Input: part model. Units: mm. Frame: model coordinates. A direction names the side the tool comes from. Round coordinates to 2 decimals unless told otherwise and drop trailing zeros. Loops run counter-clockwise (first coordinate to the right, second up) from the corner with the lowest first, then second, coordinate; pieces in that order, holes last. Notation, with made-up numbers: (29.25, 10.5) -> (87.25, 10.5) arc R11 ccw to (87.25, 21.5) -> close; hole circle Ø5 at (72, 19). An arc over 180 degrees is marked (long way). Answer as a JSON object with one key per item and string values.
```python
from build123d import *

# Parameters (mm, degrees)
F0_W      = 40.93
F0_H      = 16.6
F0_W_2    = 7.73
F0_H_2    = 7.73
F0_W_3    = 10.6
F0_H_3    = 10.6
F0_R      = 4
F0_W_4    = 6.33
F0_H_4    = 6.33
F1_DEPTH  = 2
F2_W      = 40.93
F2_H      = 16.6
F2_W_2    = 11.6
F2_H_2    = 12.6
F2_W_3    = 7.73
F2_H_3    = 7.73
F3_DEPTH  = 15
F4_W      = 40.93
F4_H      = 16.6
F4_W_2    = 11.6
F4_H_2    = 12.6
F4_W_3    = 7.73
F4_H_3    = 7.73
F5_DEPTH  = 0.5
F7_DEPTH  = 4
F8_R      = 3.5
F9_DEPTH  = 3
F10_R     = 3.5
F11_DEPTH = 3


with BuildPart() as f1:
    # F0 (on Top) → F1 (new body)
    with BuildSketch(Plane.XY):
        Rectangle(F0_W, F0_H)
        Polygon((-6.865, 6.3), (-6.865, 6.865), (6.865, 6.865), (6.865, 6.3), (18.465, 6.3), (18.465, -6.3), (6.865, -6.3), (6.865, -6.865), (-6.865, -6.865), (-6.865, -6.3), (-18.465, -6.3), (-18.465, 6.3), align=None, mode=Mode.SUBTRACT)
        Polygon((6.865, 6.865), (-6.865, 6.865), (-6.865, 6.3), (-6.865, 5.3), (-6.865, -5.3), (-6.865, -6.3), (-6.865, -6.865), (6.865, -6.865), (6.865, -6.3), (6.865, -5.3), (6.865, 5.3), (6.865, 6.3), align=None)
        Rectangle(F0_W_2, F0_H_2, mode=Mode.SUBTRACT)
        with Locations((12.165, 0)):
            Rectangle(F0_W_3, F0_H_3)
        with Locations((12.165, 0)):
            Circle(F0_R, mode=Mode.SUBTRACT)
        with Locations((-12.165, 0)):
            Rectangle(F0_W_3, F0_H_3)
        with Locations((-12.165, 0)):
            Circle(F0_R, mode=Mode.SUBTRACT)
        Rectangle(F0_W_2, F0_H_2)
        Rectangle(F0_W_4, F0_H_4, mode=Mode.SUBTRACT)
        Rectangle(F0_W_4, F0_H_4)
        Polygon((-6.865, 5.3), (-6.865, 6.3), (-18.465, 6.3), (-18.465, -6.3), (-6.865, -6.3), (-6.865, -5.3), (-17.465, -5.3), (-17.465, 5.3), align=None)
        Polygon((18.465, 6.3), (6.865, 6.3), (6.865, 5.3), (17.465, 5.3), (17.465, -5.3), (6.865, -5.3), (6.865, -6.3), (18.465, -6.3), align=None)
    extrude(amount=F1_DEPTH)

    # F2 (on face) → F3 (join)
    with BuildSketch(Plane.XY.offset(2)):
        Rectangle(F2_W, F2_H)
        with Locations((-12.665, 0)):
            Rectangle(F2_W_2, F2_H_2, mode=Mode.SUBTRACT)
        Rectangle(F2_W_3, F2_H_3, mode=Mode.SUBTRACT)
        with Locations((12.665, 0)):
            Rectangle(F2_W_2, F2_H_2, mode=Mode.SUBTRACT)
    extrude(amount=F3_DEPTH)

    # F4 (on face) → F5 (join)
    with BuildSketch(Plane.XY.offset(17)):
        Rectangle(F4_W, F4_H)
        with Locations((-12.665, 0)):
            Rectangle(F4_W_2, F4_H_2, mode=Mode.SUBTRACT)
        Rectangle(F4_W_3, F4_H_3, mode=Mode.SUBTRACT)
        with Locations((12.665, 0)):
            Rectangle(F4_W_2, F4_H_2, mode=Mode.SUBTRACT)
        Rectangle(F4_W_3, F4_H_3)
    extrude(amount=F5_DEPTH)

    # F6 (on face) → F7 (cut)
    with BuildSketch(Plane.YZ.offset(6.865)):
        Polygon((0, 9.4), (-3.4, 9.4), (-3.4, 2.6), (3.4, 2.6), (3.4, 9.4), align=None)
    extrude(amount=-F7_DEPTH, mode=Mode.SUBTRACT)

    # F8 (on face) → F9 (cut)
    with BuildSketch(Plane(origin=(0, 8.3, 0), x_dir=(-1, 0, 0), z_dir=(0, 1, 0))):
        with Locations((-12.665, 13.5)):
            Circle(F8_R)
    extrude(amount=-F9_DEPTH, mode=Mode.SUBTRACT)

    # F10 (on face) → F11 (cut)
    with BuildSketch(Plane.XZ.offset(8.3)):
        with Locations((-12.665, 13.5)):
            Circle(F10_R)
    extrude(amount=-F11_DEPTH, mode=Mode.SUBTRACT)


solid = f1.part
```
1) Section A-A, the plane y = 0. Output: boundary loops of the cut face in (x, z) (3 decimals), plus the area to 3 significant figures.
Output:
{"outline": "(-20.465, 0) -> (-16.165, 0) -> (-16.165, 2) -> (-18.465, 2) -> (-18.465, 17.5) -> (-20.465, 17.5) -> close; (-8.165, 0) -> (8.165, 0) -> (8.165, 2) -> (6.865, 2) -> (6.865, 2.6) -> (3.865, 2.6) -> (3.865, 2) -> (-3.865, 2) -> (-3.865, 17) -> (3.865, 17) -> (3.865, 9.4) -> (6.865, 9.4) -> (6.865, 17.5) -> (-6.865, 17.5) -> (-6.865, 2) -> (-8.165, 2) -> close; (16.165, 0) -> (20.465, 0) -> (20.465, 17.5) -> (18.465, 17.5) -> (18.465, 2) -> (16.165, 2) -> close", "area": "188 mm^2"}
2) Section C-C, the plane x = -2. Output: boundary loops of the cut face in (y, z) (3 decimals), plus the area to 3 significant figures.
Output:
{"outline": "(-8.3, 0) -> (8.3, 0) -> (8.3, 17.5) -> (-8.3, 17.5) -> close; hole (-3.865, 2) -> (3.865, 2) -> (3.865, 17) -> (-3.865, 17) -> close", "area": "175 mm^2"}
3) Section D-D, the plane z = 13.5. Output: boundary loops of the cut face in (x, y) (3 decimals).
Output:
{"outline": "(-20.465, -8.3) -> (-16.165, -8.3) -> (-16.165, -6.3) -> (-18.465, -6.3) -> (-18.465, 6.3) -> (-6.865, 6.3) -> (-6.865, -6.3) -> (-9.165, -6.3) -> (-9.165, -8.3) -> (20.465, -8.3) -> (20.465, 8.3) -> (16.165, 8.3) -> (16.165, 6.3) -> (18.465, 6.3) -> (18.465, -6.3) -> (6.865, -6.3) -> (6.865, 6.3) -> (9.165, 6.3) -> (9.165, 8.3) -> (-20.465, 8.3) -> close; hole (-3.865, -3.865) -> (3.865, -3.865) -> (3.865, 3.865) -> (-3.865, 3.865) -> close"}
4) Draft query along Y for faces 4 (the face through (5, -3.4, 6)), 5 (the face through (-17, 0, 2)), 6 (the face through (0, 8.3, 9)), 7 (the face through (0, 0, 0)). Return one class per face: +Y half, -Y half, draft (parallel to the pull), parting line (faces both ways), or undercut.
Output:
{"face 4": "undercut", "face 5": "undercut", "face 6": "+Y half", "face 7": "draft"}
5) Ray query, probe 1 along X at (y, z) = (4.5, 16) (3 decimals); probe 2 along X at (y, z) = (1.5, 13.5) (3 decimals); probe 3 along X at (y, z) = (2.5, 3.75) (3 decimals). Return the intervals inside material, ascending.
Output:
{"probe 1": "x = -20.465 to -18.465, -6.865 to 6.865, 18.465 to 20.465", "probe 2": "x = -20.465 to -18.465, -6.865 to -3.865, 3.865 to 6.865, 18.465 to 20.465", "probe 3": "x = -20.465 to -18.465, -6.865 to -3.865, 18.465 to 20.465"}
6) Contact query for flat-ended pins moving along their axis: P1, Ø6, axis at x = 14.5, y = 1, coming from the +Z side; P2, Ø4, axis at x = -12.665, z = 13.5, coming from the -Y side. Output: stop coordinate, or through.
Output:
{"P1": "stops at z = 2", "P2": "stops at y = 6.3"}
7) Section B-B, the plane z = 9. Output: boundary loops of the cut face in (x, y) (3 decimals).
Output:
{"outline": "(-20.465, -8.3) -> (20.465, -8.3) -> (20.465, 8.3) -> (-20.465, 8.3) -> close; hole (-18.465, -6.3) -> (-6.865, -6.3) -> (-6.865, 6.3) -> (-18.465, 6.3) -> close; hole (-3.865, -3.865) -> (3.865, -3.865) -> (3.865, -3.4) -> (6.865, -3.4) -> (6.865, -6.3) -> (18.465, -6.3) -> (18.465, 6.3) -> (6.865, 6.3) -> (6.865, 3.4) -> (3.865, 3.4) -> (3.865, 3.865) -> (-3.865, 3.865) -> close"}
8) Reachability of faces 1 (the face through (13, 6.3, 8)), 2 (the face through (11.298, -3.905, 0.986)), 3 (the face through (0, 0, 2)) from +Z, -Z, +X, -X, +Y, -Y: full face, straight path, thin tool, end or side. Return the list, or none.
Output:
{"face 1": "+Z", "face 2": "+Z, -Z", "face 3": "none"}
